```python
from build123d import *

# Parameters (mm, degrees)
SKETCH2_R           = 2.5
SKETCH2_R_2         = 2.734092972
BOSS_EXTRUDE1_DEPTH = 15
CUT_EXTRUDE1_DEPTH  = 30


with BuildPart() as part:
    # Sketch2 → Boss-Extrude1 (new body)
    with BuildSketch(Plane(origin=(0, 0, 0), x_dir=(0, 0, -1), z_dir=(1, 0, 0))):
        with BuildLine():
            Line((7.108641727, -80), (7.108641727, 0))
            ThreePointArc((7.108641727, 0), (0, 7.108641727), (-7.108641727, 0))
            Line((-7.108641727, 0), (-7.108641727, -80))
            ThreePointArc((-7.108641727, -80), (0, -87.108641727), (7.108641727, -80))
        make_face()
        with Locations((0, -80)):
            Circle(SKETCH2_R, mode=Mode.SUBTRACT)
        with BuildLine():
            Line((-0.366207439, -15.5), (0, -15.5))
            Line((0, -15.5), (0.366207439, -15.5))
            ThreePointArc((0.366207439, -15.5), (1.780421002, -16.085786438), (2.366207439, -17.5))
            Line((2.366207439, -17.5), (2.366207439, -62.5))
            ThreePointArc((2.366207439, -62.5), (1.780421002, -63.914213562), (0.366207439, -64.5))
            Line((0.366207439, -64.5), (-0.366207439, -64.5))
            ThreePointArc((-0.366207439, -64.5), (-1.780421002, -63.914213562), (-2.366207439, -62.5))
            Line((-2.366207439, -62.5), (-2.366207439, -17.5))
            ThreePointArc((-2.366207439, -17.5), (-1.780421002, -16.085786438), (-0.366207439, -15.5))
        make_face(mode=Mode.SUBTRACT)
        Circle(SKETCH2_R_2, mode=Mode.SUBTRACT)
    extrude(amount=BOSS_EXTRUDE1_DEPTH)

    # Sketch3 → Cut-Extrude1 (cut)
    with BuildSketch(Plane(origin=(0, 0, -7.108641727), x_dir=(-1, 0, 0), z_dir=(0, 0, -1))):
        with BuildLine():
            Line((-5.75, -5), (-7.5, -5))
            Line((-7.5, -5), (-7.5, -75))
            Line((-7.5, -75), (-5.75, -75))
            ThreePointArc((-5.75, -75), (-4.335786438, -74.414213562), (-3.75, -73))
            Line((-3.75, -73), (-3.75, -7))
            ThreePointArc((-3.75, -7), (-4.335786438, -5.585786438), (-5.75, -5))
        make_face()
        with BuildLine():
            Line((-7.5, -75), (-7.5, -5))
            Line((-7.5, -5), (-9.25, -5))
            ThreePointArc((-9.25, -5), (-10.664213562, -5.585786438), (-11.25, -7))
            Line((-11.25, -7), (-11.25, -73))
            ThreePointArc((-11.25, -73), (-10.664213562, -74.414213562), (-9.25, -75))
            Line((-9.25, -75), (-7.5, -75))
        make_face()
    extrude(amount=-CUT_EXTRUDE1_DEPTH, mode=Mode.SUBTRACT)


solid = part.part
```
Geometry: final body of the model. Coordinates: model frame, mm. A direction names the side the tool comes from. Round coordinates to 2 decimals unless told otherwise and drop trailing zeros. Order: outer loops, then holes, each group sorted by start corner. A loop starts at its lowest first (then second) coordinate and runs counter-clockwise, first axis right, second up. Notation, with made-up numbers: (-24.5, 64.25) -> (14.5, 64.25) arc R11 cw to (14.5, 85.25) -> close; hole circle Ø10 at (80, 64.5). An arc over 180 degrees is marked (long way). Write each question's results on one line, items separated by ' | '.
Q1. Access query for faces 4 (the face through (7, -5, 0)), 5 (the face through (0, -39, 3)), 6 (the face through (2, -40, 2.366)). Directions: +Z, -Z, +X, -X, +Y, -Y. A direction counts if a zero-diameter tool reaches every point of the face in a straight line with its end or side. Return the directions, or none.
Response values:
face 4: +Z, -Z | face 5: +Z, -Z, -X, +Y, -Y | face 6: +X, -X
Q2. Section query C-C (x = 12.75). Output: boundary loops of the cut face in (y, z).
Response values:
outline: (-80, -7.11) -> (0, -7.11) arc R7.11 ccw to (0, 7.11) -> (-80, 7.11) arc R7.11 ccw to start; hole circle Ø5 at (-80, 0); hole (-64.5, -0.37) arc R2 ccw to (-62.5, -2.37) -> (-17.5, -2.37) arc R2 ccw to (-15.5, -0.37) -> (-15.5, 0.37) arc R2 ccw to (-17.5, 2.37) -> (-62.5, 2.37) arc R2 ccw to (-64.5, 0.37) -> close; hole circle Ø5.47 at (0, 0)
Q3. Section query B-B (x = 4.75). Output: boundary loops of the cut face in (y, z), and give its area (3 significant figures).
Response values:
outline: (-80, -7.11) -> (-74.73, -7.11) -> (-74.73, 7.11) -> (-80, 7.11) arc R7.11 ccw to start; (-5.27, -7.11) -> (0, -7.11) arc R7.11 ccw to (0, 7.11) -> (-5.27, 7.11) -> close; hole circle Ø5 at (-80, 0); hole circle Ø5.47 at (0, 0) | area: 265 mm²
Q4. Pull-direction query (Z, two-part tool) for faces 1 (the face through (10.68, -74.4, -0.1)), 2 (the face through (2, -41, -7.109)), 3 (the face through (1.849, -16.07, -1.765)); classes: released by +Z, released by -Z, zero draft, split by the parting line, or undercut.
Response values:
face 1: zero draft | face 2: released by -Z | face 3: undercut
Q5. Section query A-A (y = -8.5). Output: boundary loops of the cut face in (x, z).
Response values:
outline: (0, -7.11) -> (3.75, -7.11) -> (3.75, 7.11) -> (0, 7.11) -> close; (11.25, -7.11) -> (15, -7.11) -> (15, 7.11) -> (11.25, 7.11) -> close
Q6. Ray query, line 1 along Y through (x, z) = (8.75, 0); line 2 along Z through (x, y) = (12.75, -31); line 3 along Y through (x, z) = (3.25, 0). Return the intervals inside material, ascending.
Response values:
line 1: -87.11 to -82.5, -77.5 to -75, -5 to -2.73, 2.73 to 7.11 | line 2: -7.11 to -2.37, 2.37 to 7.11 | line 3: -87.11 to -82.5, -77.5 to -64.5, -15.5 to -2.73, 2.73 to 7.11
Q7. Section query D-D (y = -22). Output: boundary loops of the cut face in (x, z).
Response values:
outline: (0, -7.11) -> (3.75, -7.11) -> (3.75, -2.37) -> (0, -2.37) -> close; (0, 2.37) -> (3.75, 2.37) -> (3.75, 7.11) -> (0, 7.11) -> close; (11.25, -7.11) -> (15, -7.11) -> (15, -2.37) -> (11.25, -2.37) -> close; (11.25, 2.37) -> (15, 2.37) -> (15, 7.11) -> (11.25, 7.11) -> close
Q8. Pin query (flat end, axial travel): pin 1 Ø1 at (y, z) = (-14, -2) entering from -X; pin 2 Ø3 at (x, z) = (7, -2.5) entering from +Y; pin 3 Ø6 at (x, z) = (3.5, 5.5) entering from -Y; pin 4 Ø1 at (x, z) = (7, -2) entering from -Y. Return the tip coordinate at first contact, or that it passes through.
Response values:
pin 1: x = 0 | pin 2: y = 7.04 | pin 3: y = -86.65 | pin 4: y = -86.95
